Check sheet for the modelled part. Datum: model origin and axes. Units: mm. A direction names the side the tool comes from. Give positions to 0.01 mm unless a question says otherwise; leave off trailing zeros. Write each loop counter-clockwise with the first axis right and the second up, starting at its lowest first coordinate (ties: lowest second). Pieces come first, ordered by that corner, then holes.
from build123d import *

# Parameters (mm, degrees)
BOX048_W                  = 45
BOX048_H                  = 36
BOX048_DEPTH              = 45
BOX049_W                  = 14
BOX049_H                  = 36
BOX049_DEPTH              = 70
CYLINDER021_R             = 20
CYLINDER021_DEPTH         = 20
FUSION014_PLACEMENT_ANGLE = 90


with BuildPart() as cube043:
    # Box048 → Box048 (new body)
    with BuildSketch(Plane.XY):
        with Locations((22.5, 18)):
            Rectangle(BOX048_W, BOX048_H)
    extrude(amount=BOX048_DEPTH)


with BuildPart() as cube044:
    # Box049 → Box049 (new body)
    with BuildSketch(Plane.XY):
        with Locations((7, 18)):
            Rectangle(BOX049_W, BOX049_H)
    extrude(amount=BOX049_DEPTH)


with BuildPart() as block:
    # Cylinder021 → Cylinder021 (new body)
    with BuildSketch(Plane(origin=(0, 18, 30), x_dir=(0, 0, 1), z_dir=(-1, 0, 0))):
        Circle(CYLINDER021_R)
    extrude(amount=CYLINDER021_DEPTH)

    # Fusion014: union Cube043, Cube044
    add(cube043.part)
    add(cube044.part)


with BuildPart() as block_1:
    # Fusion014 placement: moved
    add(block.part.moved(Location((155, -75, -70))).rotate(Axis((155, -75, -70), (0, 0, -1)), FUSION014_PLACEMENT_ANGLE))


solid = block_1.part
1) Gauge pin test, flat ends, axial feed: pin 1 (1.5 mm diameter, centred on y = -96, z = -38, fed in from -X); pin 2 (3 mm diameter, centred on x = 166, y = -113.5, fed in from +Z); pin 3 (12 mm diameter, centred on y = -93, z = -60, fed in from +X); pin 4 (1.6 mm diameter, centred on x = 154.5, z = -38, fed in from -Y). Record the tip position at first contact, or that the pin passes through.
2) Sectioned sample at C-C on y = -72.5. Record the boundary of the cut face in (x, z).
3) Sectioned sample at A-A on x = 173. Record the boundary of the cut face in (y, z).
4) Access from +Z, -Z, +X, -X, +Y, -Y to the whole of each face (thin tool, end or side, straight path). Record for faces 1 (the cylindrical face through (189.864, -65.14, -29.248)), 2 (the flat face through (173, -104, -25)), 3 (the flat face through (155, -97, -43)), 4 (the flat face through (191, -97, -43)).
5) Scan lines: L1, parallel to Z at x = 175, y = -91.5; L2, parallel to Y at x = 186.5, z = -20; L3, parallel to X at y = -87, z = -35.5. Record each from-to range of solid material in increasing order.
6) Sectioned sample at D-D on z = -40. Record the boundary of the cut face in (x, y).
7) Sectioned sample at B-B on z = -24. Record the boundary of the cut face in (x, y).
Answers below:
1. pin 1: stops at x = 155
1. pin 2: stops at z = -25
1. pin 3: stops at x = 191
1. pin 4: stops at y = -120
2. outline: circle Ø40 at (173, -40)
3. outline: (-120, -70) - (-75, -70) - (-75, -60) - (-55, -60) - (-55, -20) - (-75, -20) - (-75, 0) - (-89, 0) - (-89, -25) - (-120, -25) - close
4. face 1: +Y
4. face 2: +Z, +X, -X, -Y
4. face 3: +Z, -Z, -X, -Y
4. face 4: +Z, -Z, +X, -Y
5. L1: z = -70 to -25
5. L2: y = -89 to -75
5. L3: x = 155 to 191
6. outline: (153, -75) - (155, -75) - (155, -120) - (191, -120) - (191, -75) - (193, -75) - (193, -55) - (153, -55) - close
7. outline: (155, -89) - (191, -89) - (191, -75) - (185, -75) - (185, -55) - (161, -55) - (161, -75) - (155, -75) - close
